Autodesk Inventor part; units mm, degrees
ref_plane "YZ Plane" through (0, 0, 0) normal (1, 0, 0) x (0, 1, 0)
ref_plane "XZ Plane" through (0, 0, 0) normal (0, 1, 0) x (-1, 0, 0)
ref_plane "XY Plane" through (0, 0, 0) normal (0, 0, 1) x (1, 0, 0)
sketch "Skizze1" plane through (0, 0, 0) normal (0, 0, 1) x (1, 0, 0)
  line L0 (0, 0) -> (7.62, 0)
  line L1 (7.62, 0) -> (7.62, 3.3)
  line L2 (7.62, 3.3) -> (0, 3.3)
  line L3 (0, 3.3) -> (0, 0)
  dimension "d0" = 7.62
  dimension "d1" = 3.3
extrude "Extrusion1" add sketch "Skizze1" along normal blind 5.8
sketch "Skizze2" plane through (0, 3.3, 0) normal (0, 1, 0) x (1, 0, 0)
  line L0 (7.62, 0) -> (7.62, -5.8)
  line L1 (0, 0) -> (7.62, 0)
  line L2 (7.62, 0) -> (7.62, -1)
  line L3 (7.62, -1) -> (0, -1)
  line L4 (0, -1) -> (0, 0)
  dimension "d4" = 1
extrude "Extrusion2" add sketch "Skizze2" along normal blind 7.6
sketch "Skizze3" plane through (0, 3.3, 5.8) normal (0, 1, 0) x (1, 0, 0)
  line L0 (7.62, 4.8) -> (0, 4.8)
  line L1 (0, 4.8) -> (0, 0)
  line L2 (7.62, 0) -> (0, 0)
  line L3 (7.62, 4.8) -> (7.62, 0)
  line L4 (0.95, 2.72) -> (1.59, 2.72)
  line L5 (1.59, 2.72) -> (1.59, 2.08)
  line L6 (1.59, 2.08) -> (0.95, 2.08)
  line L7 (0.95, 2.08) -> (0.95, 2.72)
  line L8 (3.49, 2.72) -> (4.13, 2.72)
  line L9 (4.13, 2.72) -> (4.13, 2.08)
  line L10 (4.13, 2.08) -> (3.49, 2.08)
  line L11 (3.49, 2.08) -> (3.49, 2.72)
  line L12 (6.03, 2.72) -> (6.67, 2.72)
  line L13 (6.67, 2.72) -> (6.67, 2.08)
  line L14 (6.67, 2.08) -> (6.03, 2.08)
  line L15 (6.03, 2.08) -> (6.03, 2.72)
  point P0 (0, 5.8)
  dimension "d7" = 0.64
  dimension "d8" = 0.64
  dimension "d9" = 0.64
  dimension "d10" = 0.64
  dimension "d11" = 0.64
  dimension "d12" = 0.64
  dimension "d13" = 7.62
  dimension "d15" = 1.9
  dimension "d16" = 1.9
  dimension "d17" = 0.95
  dimension "d18" = 0.95
  dimension "d19" = 4.8
  dimension "d20" = 2.08
extrude "Extrusion3" add sketch "Skizze3" along normal blind 7.6 contours L4 L5 L6 L7 | L8 L9 L10 L11 | L12 L13 L14 L15
sketch "Skizze4" plane through (0, 0, 0) normal (0, -1, 0) x (1, 0, 0)
  line L0 (7.62, 0) -> (7.62, 5.8)
  line L1 (0, 5.8) -> (7.62, 5.8)
  line L2 (0, 0) -> (0, 5.8)
  line L3 (0.95, 3.72) -> (1.59, 3.72)
  line L4 (1.59, 3.72) -> (1.59, 3.08)
  line L5 (1.59, 3.08) -> (0.95, 3.08)
  line L6 (0.95, 3.08) -> (0.95, 3.72)
  line L7 (3.49, 3.72) -> (4.13, 3.72)
  line L8 (4.13, 3.72) -> (4.13, 3.08)
  line L9 (4.13, 3.08) -> (3.49, 3.08)
  line L10 (3.49, 3.08) -> (3.49, 3.72)
  line L11 (6.03, 3.72) -> (6.67, 3.72)
  line L12 (6.67, 3.72) -> (6.67, 3.08)
  line L13 (6.67, 3.08) -> (6.03, 3.08)
  line L14 (6.03, 3.08) -> (6.03, 3.72)
  dimension "d23" = 0.64
  dimension "d24" = 0.64
  dimension "d25" = 0.64
  dimension "d26" = 0.64
  dimension "d27" = 0.64
  dimension "d28" = 0.64
  dimension "d29" = 0.95
  dimension "d30" = 0.95
  dimension "d31" = 1.9
  dimension "d32" = 1.9
  dimension "d33" = 2.08
  dimension "d34" = 2.08
  dimension "d35" = 2.08
extrude "Extrusion4" add sketch "Skizze4" along normal blind 3.3
properties part number "stiftleiste"
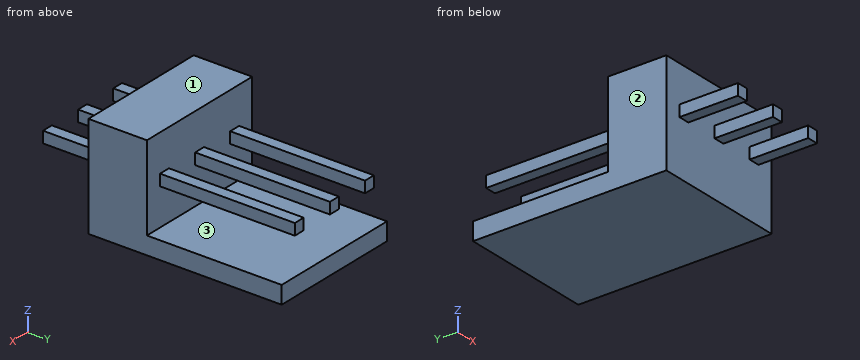
Input: part model. Units: mm. Frame: model coordinates. Face numbers are marked on the shaded views. Give positions to 0.01 mm unless a question says otherwise; leave off trailing zeros. Write each loop counter-clockwise with the first axis right and the second up, starting at its lowest first coordinate (ties: lowest second). Pieces come first, ordered by that corner, then holes.
Q1. Section A-A, the plane y = 6. Output: boundary loops of the cut face in (x, z), plus the area to 3 significant figures.
Q2. First-contact query: P1, Ø0.7, axis at y = -1.5, z = 3.5, coming from the +X side; P2, Ø1.7, axis at x = 2.5, z = 4, coming from the -Y side; P3, Ø0.5, axis at y = -2, z = 3.5, coming from the -X side. Flat tips, straight axial feed; report the tip coordinate or a pass-through.
Q3. Pull-direction query (Z, two-part tool) for the marked faces 1, 2 and 3; classes: pulls with the +Z half, pulls with the -Z half, needs draft (parallel to the pull), parting line crosses it, or undercut.
Q4. Material intervals for probe 1 along X at (y, z) = (7, 3.3); probe 2 along Z at (x, y) = (1, 6.75); probe 3 along Y at (x, z) = (1.5, 0.7), sorted ascending.
Q5. Section D-D, the plane x = 6.25. Output: boundary loops of the cut face in (y, z), plus the area to 3 significant figures.
Q6. Section B-B, the plane y = -0.75. Output: boundary loops of the cut face in (x, z).
Q7. Section C-C, the plane z = 3.3. Output: boundary loops of the cut face in (x, y).
Filled in:
1. outline: (0, 0) - (7.62, 0) - (7.62, 1) - (0, 1) - close; (0.95, 3.08) - (1.59, 3.08) - (1.59, 3.72) - (0.95, 3.72) - close; (3.49, 3.08) - (4.13, 3.08) - (4.13, 3.72) - (3.49, 3.72) - close; (6.03, 3.08) - (6.67, 3.08) - (6.67, 3.72) - (6.03, 3.72) - close
1. area: 8.85 mm2
2. P1: stops at x = 6.67
2. P2: stops at y = 0
2. P3: stops at x = 0.95
3. face 1: pulls with the +Z half
3. face 2: needs draft
3. face 3: undercut
4. probe 1: x = 0.95 to 1.59, 3.49 to 4.13, 6.03 to 6.67
4. probe 2: z = 0 to 1, 3.08 to 3.72
4. probe 3: y = 0 to 10.9
5. outline: (-3.3, 3.08) - (0, 3.08) - (0, 0) - (10.9, 0) - (10.9, 1) - (3.3, 1) - (3.3, 3.08) - (10.9, 3.08) - (10.9, 3.72) - (3.3, 3.72) - (3.3, 5.8) - (0, 5.8) - (0, 3.72) - (-3.3, 3.72) - close
5. area: 33.7 mm2
6. outline: (0.95, 3.08) - (1.59, 3.08) - (1.59, 3.72) - (0.95, 3.72) - close; (3.49, 3.08) - (4.13, 3.08) - (4.13, 3.72) - (3.49, 3.72) - close; (6.03, 3.08) - (6.67, 3.08) - (6.67, 3.72) - (6.03, 3.72) - close
7. outline: (0, 0) - (0.95, 0) - (0.95, -3.3) - (1.59, -3.3) - (1.59, 0) - (3.49, 0) - (3.49, -3.3) - (4.13, -3.3) - (4.13, 0) - (6.03, 0) - (6.03, -3.3) - (6.67, -3.3) - (6.67, 0) - (7.62, 0) - (7.62, 3.3) - (6.67, 3.3) - (6.67, 10.9) - (6.03, 10.9) - (6.03, 3.3) - (4.13, 3.3) - (4.13, 10.9) - (3.49, 10.9) - (3.49, 3.3) - (1.59, 3.3) - (1.59, 10.9) - (0.95, 10.9) - (0.95, 3.3) - (0, 3.3) - close
